Check sheet for the modelled part. Datum: model origin and axes. Units: mm. A direction names the side the tool comes from. Round coordinates to 2 decimals unless told otherwise and drop trailing zeros. Order: outer loops, then holes, each group sorted by start corner. A loop starts at its lowest first (then second) coordinate and runs counter-clockwise, first axis right, second up.
Q1. Scan lines: probe 1 along Y at (x, z) = (12.7, 2.75); probe 2 along Y at (x, z) = (11, 2.25); probe 3 along Y at (x, z) = (190.5, 2.75). Record each from-to range of solid material in increasing order.
Q2. Mould release check, pull along X, two halves, no side actions. Record for faces 3 (the cylindrical face through (111.762, 12.812, 3.219)), 4 (the flat face through (228.6, 26, 3)), 5 (the flat face through (216, 50.8, 3)): +X half, -X half, draft (parallel to the pull), parting line (faces both ways), or undercut.
Q3. Cross-section at C-C on z = 1. Give the number of separate pieces and of enclosed holes in the cut face, then the cut area to 3 significant figures.
Q4. Cross-section at B-B on x = 88.9. Record the cut outline in (y, z), then the cut area to 3 significant figures.
Q5. Cross-section at D-D on x = 215.9. Record the cut outline in (y, z).
Q6. Depth check by flat-ended pin: P1, Ø3, axis at x = 83.5, z = 2, coming from the +Y side. Enter the tip coordinate at first touch or a pass-through.
Q7. Set-up check for faces 1 (the flat face through (203.2, 38, 3)), 2 (the flat face through (116, 20, 0)): record each of +Z, -Z, +X, -X, +Y, -Y from which the full face is reachable in a straight line by a thin tool's end or side.
Q8. Cross-section at A-A on y = 38.1. Record the cut outline in (x, z), then the cut area to 3 significant figures.
from build123d import *

# Parameters (mm, degrees)
BOSS_EXTRUDE1_DEPTH = 6.35
SKETCH2_R           = 2.54
CUT_EXTRUDE1_DEPTH  = 235.26250767


with BuildPart() as part:
    # Sketch1 → Boss-Extrude1 (new body)
    with BuildSketch(Plane.XY):
        Polygon((0, 0), (0, 50.8), (25.4, 50.8), (25.4, 25.4), (203.2, 25.4), (203.2, 50.8), (228.6, 50.8), (228.6, 0), align=None)
    extrude(amount=BOSS_EXTRUDE1_DEPTH)

    # Sketch2 → Cut-Extrude1 (cut, through all)
    with BuildSketch(Plane.XY.offset(6.35)):
        with Locations((12.7, 38.1)):
            Circle(SKETCH2_R)
        with Locations((12.7, 12.7)):
            Circle(SKETCH2_R)
        with Locations((38.1, 12.7)):
            Circle(SKETCH2_R)
        with Locations((63.5, 12.7)):
            Circle(SKETCH2_R)
        with Locations((88.9, 12.7)):
            Circle(SKETCH2_R)
        with Locations((114.3, 12.7)):
            Circle(SKETCH2_R)
        with Locations((139.7, 12.7)):
            Circle(SKETCH2_R)
        with Locations((165.1, 12.7)):
            Circle(SKETCH2_R)
        with Locations((190.5, 12.7)):
            Circle(SKETCH2_R)
        with Locations((215.9, 12.7)):
            Circle(SKETCH2_R)
        with Locations(Location((215.9, 38.1, 0), (0, 0, 180))):
            Circle(SKETCH2_R)
    extrude(amount=-CUT_EXTRUDE1_DEPTH, mode=Mode.SUBTRACT)


solid = part.part
Results found:
1. probe 1: y = 0 to 10.16, 15.24 to 35.56, 40.64 to 50.8
1. probe 2: y = 0 to 10.81, 14.59 to 36.21, 39.99 to 50.8
1. probe 3: y = 0 to 10.16, 15.24 to 25.4
2. face 3: undercut
2. face 4: +X half
2. face 5: draft
3. separate pieces: 1
3. enclosed holes: 11
3. area: 6,870 mm2
4. outline: (0, 0) - (10.16, 0) - (10.16, 6.35) - (0, 6.35) - close; (15.24, 0) - (25.4, 0) - (25.4, 6.35) - (15.24, 6.35) - close
4. area: 129 mm2
5. outline: (0, 0) - (10.16, 0) - (10.16, 6.35) - (0, 6.35) - close; (15.24, 0) - (35.56, 0) - (35.56, 6.35) - (15.24, 6.35) - close; (40.64, 0) - (50.8, 0) - (50.8, 6.35) - (40.64, 6.35) - close
6. P1: stops at y = 25.4
7. face 1: +Z, -Z, +Y
7. face 2: -Z, +X, -X, +Y, -Y
8. outline: (0, 0) - (10.16, 0) - (10.16, 6.35) - (0, 6.35) - close; (15.24, 0) - (25.4, 0) - (25.4, 6.35) - (15.24, 6.35) - close; (203.2, 0) - (213.36, 0) - (213.36, 6.35) - (203.2, 6.35) - close; (218.44, 0) - (228.6, 0) - (228.6, 6.35) - (218.44, 6.35) - close
8. area: 258 mm2
